```python
from build123d import *

# Parameters (mm, degrees)
SKETCH1_R             = 1.7
BOSS_EXTRUDE1_DEPTH   = 5
SKETCH3_W             = 60
SKETCH3_H             = 35
SKETCH3_R             = 4.5
SKETCH3_R_2           = 2.5
BOSS_EXTRUDE2_DEPTH   = 5
SKETCH4_R             = 3
CUT_EXTRUDE1_DEPTH    = 3
SKETCH11_R            = 2.35
SKETCH11_R_2          = 1.7
BOSS_EXTRUDE3_DEPTH   = 4
BOSS_EXTRUDE3_2_DEPTH = 4
SKETCH12_R            = 2.658625551
SKETCH12_R_2          = 1.7
SKETCH12_R_3          = 2.826964015
BOSS_EXTRUDE4_DEPTH   = 5
CHAMFER1_SIZE         = 15
BOSS_EXTRUDE5_DEPTH   = 3
BOSS_EXTRUDE6_DEPTH   = 3
CHAMFER2_SIZE         = 2
CHAMFER2_SIZE2        = 1


with BuildPart() as part:
    # Sketch1 → Boss-Extrude1 (new body)
    # profile 1 of 4: a face of its own
    with BuildSketch(Plane.XY):
        Polygon((111.623766163, 210.92362241), (111.623766163, 235.92362241), (96.623766163, 235.92362241), (91.623766163, 235.92362241), (91.623766163, 225.92362241), (91.623766163, 215.92362241), (91.623766163, 210.92362241), (96.623766163, 210.92362241), align=None)
        with Locations((96.623766163, 215.92362241)):
            Circle(SKETCH1_R, mode=Mode.SUBTRACT)
        with Locations((96.623766163, 225.92362241)):
            Circle(SKETCH1_R, mode=Mode.SUBTRACT)
    # profile 2 of 4: a face of its own
    with BuildSketch(Plane.XY):
        Polygon((126.623766163, 235.92362241), (111.623766163, 235.92362241), (111.623766163, 210.92362241), (126.623766163, 210.92362241), (131.623766163, 210.92362241), (131.623766163, 215.92362241), (131.623766163, 225.92362241), (131.623766163, 235.92362241), align=None)
        with Locations((126.623766163, 215.92362241)):
            Circle(SKETCH1_R, mode=Mode.SUBTRACT)
        with Locations((126.623766163, 225.92362241)):
            Circle(SKETCH1_R, mode=Mode.SUBTRACT)
    # profile 3 of 4: a face of its own
    with BuildSketch(Plane.XY):
        Polygon((91.623766163, 225.92362241), (91.623766163, 235.92362241), (81.623766163, 235.92362241), (81.623766163, 210.92362241), (91.623766163, 210.92362241), (91.623766163, 215.92362241), align=None)
    # profile 4 of 4: a face of its own
    with BuildSketch(Plane.XY):
        Polygon((141.623766163, 235.92362241), (131.623766163, 235.92362241), (131.623766163, 225.92362241), (131.623766163, 215.92362241), (131.623766163, 210.92362241), (141.623766163, 210.92362241), align=None)
    extrude(amount=BOSS_EXTRUDE1_DEPTH)

    # Sketch3 → Boss-Extrude2 (add)
    with BuildSketch(Plane(origin=(0, 235.92362241, 0), x_dir=(1, 0, 0), z_dir=(0, 1, 0))):
        with Locations((111.623766163, -22.5)):
            Rectangle(SKETCH3_W, SKETCH3_H)
        with Locations(Location((111.623766163, -25.961896785, 0), (0, 0, 180))):
            Circle(SKETCH3_R, mode=Mode.SUBTRACT)
        with Locations(Location((129.873766163, -25.961896785, 0), (0, 0, 180))):
            Circle(SKETCH3_R_2, mode=Mode.SUBTRACT)
        with Locations(Location((93.373766163, -25.961896785, 0), (0, 0, 180))):
            Circle(SKETCH3_R_2, mode=Mode.SUBTRACT)
    extrude(amount=-BOSS_EXTRUDE2_DEPTH)

    # Sketch4 → Cut-Extrude1 (cut)
    with BuildSketch(Plane.XY.offset(5)):
        with Locations((126.623766163, 215.92362241)):
            Circle(SKETCH4_R)
        with Locations((126.623766163, 225.92362241)):
            Circle(SKETCH4_R)
        with Locations((96.623766163, 225.92362241)):
            Circle(SKETCH4_R)
        with Locations((96.623766163, 215.92362241)):
            Circle(SKETCH4_R)
    extrude(amount=-CUT_EXTRUDE1_DEPTH, mode=Mode.SUBTRACT)



with BuildPart() as body_2:
    # Sketch11 → Boss-Extrude3 (new body)
    with BuildSketch(Plane.XZ.offset(-230.92362241)):
        with Locations((129.873766163, 25.961896785)):
            Circle(SKETCH11_R)
        with Locations((129.873766163, 25.961896785)):
            Circle(SKETCH11_R_2, mode=Mode.SUBTRACT)
    extrude(amount=BOSS_EXTRUDE3_DEPTH)


with BuildPart() as body_3:
    # Sketch11 → Boss-Extrude3 2 (new body)
    with BuildSketch(Plane.XZ.offset(-230.92362241)):
        with Locations((93.373766163, 25.961896785)):
            Circle(SKETCH11_R)
        with Locations((93.373766163, 25.961896785)):
            Circle(SKETCH11_R_2, mode=Mode.SUBTRACT)
    extrude(amount=BOSS_EXTRUDE3_2_DEPTH)


with BuildPart() as part_1:
    add(part.part)

    add(body_2.part)  # Boss-Extrude4 merges body 2

    add(body_3.part)  # Boss-Extrude4 merges body 3
    # Sketch12 → Boss-Extrude4 (add)
    # profile 1 of 2: a face of its own
    with BuildSketch(Plane(origin=(0, 230.92362241, 0), x_dir=(1, 0, 0), z_dir=(0, 1, 0))):
        with Locations((129.873766163, -25.961896785)):
            Circle(SKETCH12_R)
        with Locations((129.873766163, -25.961896785)):
            Circle(SKETCH12_R_2, mode=Mode.SUBTRACT)
    # profile 2 of 2: a face of its own
    with BuildSketch(Plane(origin=(0, 230.92362241, 0), x_dir=(1, 0, 0), z_dir=(0, 1, 0))):
        with Locations((93.373766163, -25.961896785)):
            Circle(SKETCH12_R_3)
        with Locations((93.373766163, -25.961896785)):
            Circle(SKETCH12_R_2, mode=Mode.SUBTRACT)
    extrude(amount=BOSS_EXTRUDE4_DEPTH)

    # Chamfer1
    chamfer1_edges = [part_1.edges().sort_by_distance(p)[0] for p in [
        (141.623766163, 233.42362241, 40),
        (81.623766163, 233.42362241, 40),
    ]]
    chamfer(chamfer1_edges, length=CHAMFER1_SIZE)

    # Sketch13 → Boss-Extrude5 (add)
    with BuildSketch(Plane.ZY.offset(-81.623766163)):
        Polygon((25, 230.92362241), (5, 210.92362241), (5, 230.92362241), align=None)
        Polygon((5, 210.92362241), (5, 230.92362241), (25, 230.92362241), (25, 235.92362241), (0, 235.92362241), (0, 210.92362241), align=None)
    extrude(amount=-BOSS_EXTRUDE5_DEPTH)

    # Sketch14 → Boss-Extrude6 (add)
    with BuildSketch(Plane(origin=(141.623766163, 0, 0), x_dir=(0, 0, -1), z_dir=(1, 0, 0))):
        Polygon((-5, 210.92362241), (-25, 230.92362241), (-5, 230.92362241), align=None)
        Polygon((0, 210.92362241), (0, 235.92362241), (-25, 235.92362241), (-25, 230.92362241), (-5, 230.92362241), (-5, 210.92362241), align=None)
    extrude(amount=-BOSS_EXTRUDE6_DEPTH)

    # Chamfer2
    chamfer2_edges = [part_1.edges().sort_by_distance(p)[0] for p in [
        (91.023766163, 230.92362241, 25.961896785),
        (127.523766163, 230.92362241, 25.961896785),
    ]]
    chamfer2_side = [part_1.faces().sort_by_distance(p)[0] for p in [
        (111.623766163, 230.92362241, 21.140138657),
    ]]
    chamfer(chamfer2_edges, length=CHAMFER2_SIZE, length2=CHAMFER2_SIZE2, reference=chamfer2_side[0])


solid = part_1.part
```
Could you check a few things on this model? Use its own coordinates, in mm. A direction names the side the tool comes from. Give positions to 0.01 mm unless a question says otherwise; leave off trailing zeros. Order: outer loops, then holes, each group sorted by start corner. A loop starts at its lowest first (then second) coordinate and runs counter-clockwise, first axis right, second up.
Q1. If I drill on line 1 along X through (y, z) = (224, 14.5); line 2 along X through (y, z) = (227, 3.5); line 3 along Y through (x, z) = (114, 31), over which ranges is the centre line in solid material (lowest first)?
Q2. Suppose I cut it at C-C, the plane x = 121. Write out the boundary of the cut face in (y, z), and give its area (3 significant figures).
Q3. We'd pull the mould along X, two halves only. Please class faces 5 (the cylindrical face through (92.025, 231.361, 26.996)), 6 (the flat face through (141.624, 226, 10)), 7 (the flat face through (128, 226.924, 27)): +X half, -X half, draft (parallel to the pull), parting line (faces both ways), or undercut.
Q4. I'm going to push flat-ended pins straight in: P1, Ø3, axis at x = 123.5, y = 226, coming from the +Z side; P2, Ø5.5, axis at x = 126.62, y = 225.92, coming from the +Z side; P3, Ø2.5, axis at x = 96.62, y = 225.92, coming from the +Z side; P4, Ø12, axis at x = 104, z = 21, coming from the -Y side. Where does each tip first touch, or does it pass through?
Q5. Suppose I cut it at D-D, the plane z = 12. Write out the boundary of the cut face in (x, y), and give its area (3 significant figures).
Q6. Suppose I cut it at B-B, the plane z = 16. Write out the boundary of the cut face in (x, y).
Q7. For faces 1 (the flat face through (111, 230.924, 18)), 2 (the flat face through (134.019, 233.459, 32.605)), 3 (the flat face through (97, 214, 2)), 4 (the flat face through (95, 226.924, 27)), which set-ups out of +Z, -Z, +X, -X, +Y, -Y let a thin tool reach every point of the face, with its end or its side?
Q8. Suppose I cut it at A-A, the plane y = 233. Write out the boundary of the cut face in (x, z).
Solution:
1. line 1: x = 81.62 to 84.62, 138.62 to 141.62
1. line 2: x = 81.62 to 93.82, 99.42 to 123.82, 129.42 to 141.62
1. line 3: y = 230.92 to 235.92
2. outline: (210.92, 0) - (235.92, 0) - (235.92, 40) - (230.92, 40) - (230.92, 5) - (210.92, 5) - close
2. area: 300 mm2
3. face 5: undercut
3. face 6: +X half
3. face 7: draft
4. P1: stops at z = 5
4. P2: stops at z = 28.21
4. P3: passes through
4. P4: stops at y = 230.92
5. outline: (81.62, 217.92) - (84.62, 217.92) - (84.62, 230.92) - (138.62, 230.92) - (138.62, 217.92) - (141.62, 217.92) - (141.62, 235.92) - (81.62, 235.92) - close
5. area: 378 mm2
6. outline: (81.62, 221.92) - (84.62, 221.92) - (84.62, 230.92) - (138.62, 230.92) - (138.62, 221.92) - (141.62, 221.92) - (141.62, 235.92) - (81.62, 235.92) - close
7. face 1: -Y
7. face 2: +Z, +X, +Y, -Y
7. face 3: +Z
7. face 4: +Z, +X, -X, -Y
8. outline: (81.62, 0) - (141.62, 0) - (141.62, 25) - (126.62, 40) - (96.62, 40) - (81.62, 25) - close; hole circle Ø3.4 at (93.37, 25.96); hole circle Ø9 at (111.62, 25.96); hole circle Ø3.4 at (129.87, 25.96)
